Design review of the part built by this model. Coordinates are the model's own, in mm. Face numbers are marked on the shaded views. A direction names the side the tool comes from. Give positions to 0.01 mm unless a question says otherwise; leave off trailing zeros. Loops run counter-clockwise (first coordinate to the right, second up) from the corner with the lowest first, then second, coordinate; pieces in that order, holes last.
from build123d import *

# Parameters (mm, degrees)
F1_DEPTH = 8
F3_DEPTH = 25
F4_R     = 5
F5_DEPTH = 0.4


with BuildPart() as f1:
    # F0 (on Top) → F1 (new body)
    with BuildSketch(Plane.XY):
        with BuildLine():
            Line((-1, 0), (0, 0))
            Line((0, 0), (5, 0))
            Line((5, 0), (5, 14))
            Line((5, 14), (-18, 14))
            Line((-18, 14), (-18, 9))
            Line((-18, 9), (0, 9))
            Line((0, 9), (0, 3))
            Line((0, 3), (-1, 3))
            ThreePointArc((-1, 3), (-2.5, 1.5), (-1, 0))
        make_face()
    extrude(amount=F1_DEPTH)

    # F2 (on face) → F3 (cut)
    with BuildSketch(Plane(origin=(0, 14, 0), x_dir=(-1, 0, 0), z_dir=(0, 1, 0))):
        with BuildLine():
            ThreePointArc((15, 2.5), (16.0606601718, 2.9393398282), (16.5, 4))
            ThreePointArc((16.5, 4), (16.0606601718, 5.0606601718), (15, 5.5))
            Line((15, 5.5), (15, 5.4696938457))
            ThreePointArc((15, 5.4696938457), (15.8618950039, 4.9486832981), (16.2, 4))
            ThreePointArc((16.2, 4), (15.8618950039, 3.0513167019), (15, 2.5303061543))
            Line((15, 2.5303061543), (15, 2.5))
        make_face()
        with BuildLine():
            ThreePointArc((15, 5.4696938457), (14.9252882939, 5.4829852274), (14.85, 5.4924811557))
            ThreePointArc((14.85, 5.4924811557), (13.5, 4), (14.85, 2.5075188443))
            ThreePointArc((14.85, 2.5075188443), (14.9252882939, 2.5170147726), (15, 2.5303061543))
            Line((15, 2.5303061543), (15, 5.4696938457))
        make_face()
        with BuildLine():
            ThreePointArc((14.85, 2.5075188443), (13.5, 4), (14.85, 5.4924811557))
            ThreePointArc((14.85, 5.4924811557), (14.7750941626, 5.4981191097), (14.7, 5.5))
            ThreePointArc((14.7, 5.5), (13.2, 4), (14.7, 2.5))
            ThreePointArc((14.7, 2.5), (14.7750941626, 2.5018808903), (14.85, 2.5075188443))
        make_face()
        with BuildLine():
            ThreePointArc((16.2, 4), (15.8618950039, 4.9486832981), (15, 5.4696938457))
            Line((15, 5.4696938457), (15, 2.5303061543))
            ThreePointArc((15, 2.5303061543), (15.8618950039, 3.0513167019), (16.2, 4))
        make_face()
        with BuildLine():
            Line((15, 5.4696938457), (15, 5.5))
            ThreePointArc((15, 5.5), (14.9249058374, 5.4981191097), (14.85, 5.4924811557))
            ThreePointArc((14.85, 5.4924811557), (14.9252882939, 5.4829852274), (15, 5.4696938457))
        make_face()
        with BuildLine():
            ThreePointArc((14.85, 2.5075188443), (14.9249058374, 2.5018808903), (15, 2.5))
            Line((15, 2.5), (15, 2.5303061543))
            ThreePointArc((15, 2.5303061543), (14.9252882939, 2.5170147726), (14.85, 2.5075188443))
        make_face()
        with BuildLine():
            ThreePointArc((14.85, 5.4924811557), (14.9249058374, 5.4981191097), (15, 5.5))
            Line((15, 5.5), (14.7, 5.5))
            ThreePointArc((14.7, 5.5), (14.7750941626, 5.4981191097), (14.85, 5.4924811557))
        make_face()
        with BuildLine():
            Line((14.7, 2.5), (15, 2.5))
            ThreePointArc((15, 2.5), (14.9249058374, 2.5018808903), (14.85, 2.5075188443))
            ThreePointArc((14.85, 2.5075188443), (14.7750941626, 2.5018808903), (14.7, 2.5))
        make_face()
    extrude(amount=-F3_DEPTH, mode=Mode.SUBTRACT)

    # F4
    f4_edges = [f1.edges().sort_by_distance(p)[0] for p in [
        (5, 14, 4),
        (5, 0, 4),
    ]]
    fillet(f4_edges, radius=F4_R)

    # F5 (add): a face of the model
    f5_faces = [f1.faces().sort_by_distance(p)[0] for p in [
        (-18, 11.5, 4),
    ]]
    extrude(f5_faces, amount=F5_DEPTH)


solid = f1.part
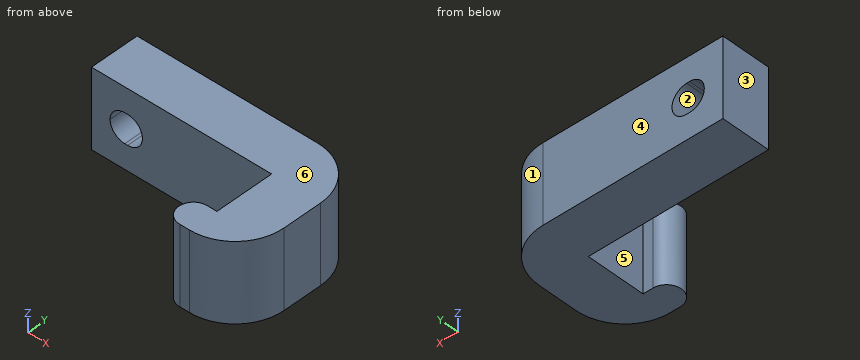
Q1. Insertion check: pin 1 (4 mm diameter, centred on x = -3.5, z = 2.5, fed in from -Y); pin 2 (1.8 mm diameter, centred on y = 7, z = 5.5, fed in from -X); pin 3 (8 mm diameter, centred on x = -0.5, y = 2, fed in from -Z). Each pin has a flat end and moves straight along its axis. Give the tip position at first contact, or say it passes through.
Results:
pin 1: stops at y = 0.09
pin 2: stops at x = 0
pin 3: stops at z = 0
Q2. Draft analysis for pull direction X (two halves, no side actions). For the marked faces 1, 2, 3 and 4, state which applies: pulls with the +X half, pulls with the -X half, needs draft (parallel to the pull), parting line crosses it, or undercut.
Results:
face 1: pulls with the +X half
face 2: undercut
face 3: pulls with the -X half
face 4: needs draft
Q3. Take a section at A-A (y = 13). Give the boundary of the cut face in (x, z), plus the area to 3 significant figures.
Results:
outline: (-18.4, 0) - (3, 0) - (3, 8) - (-18.4, 8) - close; hole (-15, 2.5) - (-14.7, 2.5) arc R1.5 ccw to (-14.7, 5.5) - (-15, 5.5) arc R1.5 ccw to start
area: 163 mm2
Q4. Wall thickness on line 1 (Y direction, x = -15.5, z = 0.5); line 2 (X direction, y = 5.75, z = 3); line 3 (Y direction, x = -2, z = 3.75): over which ranges is each line inside the solid? List them lowest first.
Results:
line 1: y = 9 to 14
line 2: x = 0 to 5
line 3: y = 0.38 to 2.62, 9 to 14
Q5. Tool access review of the marked faces 5 and 6: name each direction out of +Z, -Z, +X, -X, +Y, -Y from which nothing blocks a thin tool from reaching the whole face with its end or side.
Results:
face 5: +Z, -Z, -X
face 6: +Z, +X, -X, +Y, -Y
Q6. Take a section at B-B (z = 4.5). Give the boundary of the cut face in (x, y), plus the area to 3 significant figures.
Results:
outline: (-18.4, 9) - (-16.41, 9) - (-16.41, 14) - (-18.4, 14) - close; (-13.29, 9) - (0, 9) - (0, 3) - (-1, 3) arc R1.5 ccw to (-1, 0) - (0, 0) arc R5 ccw to (5, 5) - (5, 9) arc R5 ccw to (0, 14) - (-13.29, 14) - close
area: 142 mm2
Q7. Take a section at C-C (z = 6.75). Give the boundary of the cut face in (x, y), plus the area to 3 significant figures.
Results:
outline: (-18.4, 9) - (0, 9) - (0, 3) - (-1, 3) arc R1.5 ccw to (-1, 0) - (0, 0) arc R5 ccw to (5, 5) - (5, 9) arc R5 ccw to (0, 14) - (-18.4, 14) - close
area: 158 mm2
Q8. Take a section at D-D (y = 10). Give the boundary of the cut face in (x, z).
Results:
outline: (-18.4, 0) - (4.9, 0) - (4.9, 8) - (-18.4, 8) - close; hole (-15, 2.5) - (-14.7, 2.5) arc R1.5 ccw to (-14.7, 5.5) - (-15, 5.5) arc R1.5 ccw to start
